Model file for the job. Use its own axes, mm. Face numbers are marked on the shaded views. A direction names the side the tool comes from. Round coordinates to 2 decimals unless told otherwise and drop trailing zeros. Order: outer loops, then holes, each group sorted by start corner. A loop starts at its lowest first (then second) coordinate and runs counter-clockwise, first axis right, second up. Notation, with made-up numbers: (85, 58) - (115, 58) arc R6 ccw to (115, 62) - close; hole circle Ø8 at (-8, 48.25). An arc over 180 degrees is marked (long way). Write item = value, one per line.
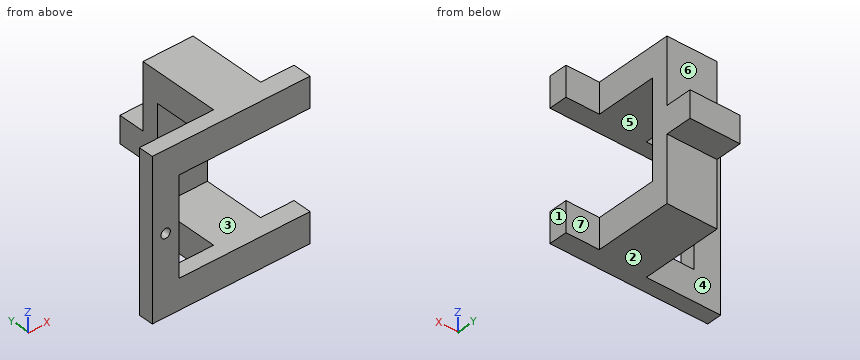
```python
from build123d import *

# Parameters (mm, degrees)
BOSS_EXTRUDE1_DEPTH = 47
SKETCH2_W           = 8
SKETCH2_H           = 8
BOSS_EXTRUDE2_DEPTH = 15
SKETCH4_W           = 29
SKETCH4_H           = 18.42
CUT_EXTRUDE4_DEPTH  = 15
SKETCH5_W           = 29
SKETCH5_H           = 5.58
CUT_EXTRUDE5_DEPTH  = 39.25
SKETCH7_R           = 1.4
CUT_EXTRUDE6_DEPTH  = 39.25


with BuildPart() as part:
    # Sketch1 → Boss-Extrude1 (new body)
    with BuildSketch(Plane.XY):
        Polygon((-6.810719807, 3.369565217), (-6.810719807, -21.130434783), (-29.058309823, -21.130434783), (-29.058309823, -25.630434783), (18.189280193, -25.630434783), (18.189280193, -20.050434783), (8.189280193, -20.050434783), (8.189280193, 3.369565217), align=None)
    extrude(amount=BOSS_EXTRUDE1_DEPTH)

    # Sketch2 → Boss-Extrude2 (add)
    with BuildSketch(Plane(origin=(8.189280193, 0, 0), x_dir=(0, 0, -1), z_dir=(1, 0, 0))):
        with Locations((-23.5, 7.369565217)):
            Rectangle(SKETCH2_W, SKETCH2_H)
    extrude(amount=-BOSS_EXTRUDE2_DEPTH)

    # Sketch4 → Cut-Extrude4 (cut)
    with BuildSketch(Plane(origin=(8.189280193, 0, 0), x_dir=(0, 0, -1), z_dir=(1, 0, 0))):
        with Locations((-23.5, -10.840434783)):
            Rectangle(SKETCH4_W, SKETCH4_H)
    extrude(amount=-CUT_EXTRUDE4_DEPTH, mode=Mode.SUBTRACT)

    # Sketch5 → Cut-Extrude5 (cut)
    with BuildSketch(Plane(origin=(18.189280193, 0, 0), x_dir=(0, 0, -1), z_dir=(1, 0, 0))):
        with Locations((-23.5, -22.840434783)):
            Rectangle(SKETCH5_W, SKETCH5_H)
    extrude(amount=-CUT_EXTRUDE5_DEPTH, mode=Mode.SUBTRACT)

    # Sketch7 → Cut-Extrude6 (cut)
    with BuildSketch(Plane(origin=(0, -21.130434783, 0), x_dir=(1, 0, 0), z_dir=(0, 1, 0))):
        with Locations((-25.059514815, -23.5)):
            Circle(SKETCH7_R)
    extrude(amount=-CUT_EXTRUDE6_DEPTH, mode=Mode.SUBTRACT)


solid = part.part
```
1) Wall check: line 1 along Z through (x, y) = (-6.5, -23.5); line 2 along X through (y, z) = (-22.1, 23.5); line 3 along Y through (x, z) = (-4, 39). Give the ranges that are in metal, low to high.
Conclusion:
line_1 = 0 to 9, 38 to 47
line_2 = -29.06 to -26.46, -23.66 to -21.06
line_3 = -25.63 to 3.37
2) 3-axis set-ups, long thin cutter, end or side, ignore diameter. For the marked faces 4, 5, 6 and 7: which of +Z, -Z, +X, -X, +Y, -Y reach the whole face in a straight line?
Conclusion:
face_4 = +Z, -Z, -X, +Y
face_5 = +X, -Y
face_6 = +Z, +X, -X, +Y
face_7 = +Z, -Z, +X, +Y
3) Mould opens along Z. For the marked faces 1, 2 and 3 say: +Z half, -Z half, draft (parallel to the pull), parting line (faces both ways), or undercut.
Conclusion:
face_1 = draft
face_2 = -Z half
face_3 = undercut
4) Flat gauge pins, fed straight in: pin 1 Ø18 at (x, z) = (-17, 33) entering from +Y; pin 2 Ø9 at (x, y) = (4, 8) entering from +Z; pin 3 Ø3 at (x, z) = (4.5, 19) entering from -Y. Where does each tip first touch, or does it go through?
Conclusion:
pin_1 = -21.13
pin_2 = 27.5
pin_3 = -1.63
5) Cut at C-C (x = -6). Write the cut outline in (y, z).
Conclusion:
outline = (-25.63, 0) - (3.37, 0) - (3.37, 19.5) - (11.37, 19.5) - (11.37, 27.5) - (3.37, 27.5) - (3.37, 47) - (-25.63, 47) - (-25.63, 38) - (-1.63, 38) - (-1.63, 9) - (-25.63, 9) - close
6) Cut at A-A (z = 12). Write the cut outline in (x, y), and give its area (3 significant figures).
Conclusion:
outline = (-29.06, -25.63) - (-21.06, -25.63) - (-21.06, -21.13) - (-29.06, -21.13) - close; (-6.81, -1.63) - (8.19, -1.63) - (8.19, 3.37) - (-6.81, 3.37) - close
area = 111 mm^2
7) Cut at D-D (z = 23.5). Write the cut outline in (x, y), and give its area (3 significant figures).
Conclusion:
outline = (-29.06, -25.63) - (-26.46, -25.63) - (-26.46, -21.13) - (-29.06, -21.13) - close; (-23.66, -25.63) - (-21.06, -25.63) - (-21.06, -21.13) - (-23.66, -21.13) - close; (-6.81, -1.63) - (8.19, -1.63) - (8.19, 11.37) - (-6.81, 11.37) - close
area = 218 mm^2
8) Cut at B-B (y = -19). Write the cut outline in (x, z).
Conclusion:
outline = (-6.81, 0) - (8.19, 0) - (8.19, 9) - (-6.81, 9) - close; (-6.81, 38) - (8.19, 38) - (8.19, 47) - (-6.81, 47) - close
